```python
from build123d import *

# Parameters (mm, degrees)
SKETCH1_W           = 230
SKETCH1_H           = 90
SKETCH1_R           = 5
SKETCH1_R_2         = 3.5
SKETCH1_R_3         = 2.25
SKETCH1_W_2         = 40
SKETCH1_H_2         = 10
SKETCH1_H_3         = 7
BOSS_EXTRUDE1_DEPTH = 6
SKETCH2_W           = 230
SKETCH2_H           = 6
BOSS_EXTRUDE2_DEPTH = 12
CUT_EXTRUDE1_REACH  = 145.544
SKETCH3_R           = 2.25


with BuildPart() as part:
    # Sketch1 → Boss-Extrude1 (new body)
    with BuildSketch(Plane(origin=(0, 0, 0), x_dir=(1, 0, 0), z_dir=(0, 1, 0))):
        Rectangle(SKETCH1_W, SKETCH1_H)
        with Locations(Location((0, 0, 0), (0, 0, 270))):
            Circle(SKETCH1_R, mode=Mode.SUBTRACT)
        with Locations(Location((0, 22.25, 0), (0, 0, 270))):
            Circle(SKETCH1_R_2, mode=Mode.SUBTRACT)
        with Locations(Location((0, -22.25, 0), (0, 0, 90))):
            Circle(SKETCH1_R_2, mode=Mode.SUBTRACT)
        with Locations(Location((110, 40, 0), (0, 0, 270))):
            Circle(SKETCH1_R_3, mode=Mode.SUBTRACT)
        with Locations(Location((110, -32.5, 0), (0, 0, 270))):
            Circle(SKETCH1_R_3, mode=Mode.SUBTRACT)
        with Locations(Location((-110, 40, 0), (0, 0, 90))):
            Circle(SKETCH1_R_3, mode=Mode.SUBTRACT)
        with Locations(Location((-110, -32.5, 0), (0, 0, 90))):
            Circle(SKETCH1_R_3, mode=Mode.SUBTRACT)
        with Locations((55, 0)):
            Rectangle(SKETCH1_W_2, SKETCH1_H_2, mode=Mode.SUBTRACT)
        with Locations((55, 22.25)):
            Rectangle(SKETCH1_W_2, SKETCH1_H_3, mode=Mode.SUBTRACT)
        with Locations((55, -22.25)):
            Rectangle(SKETCH1_W_2, SKETCH1_H_3, mode=Mode.SUBTRACT)
        with Locations((-55, -22.25)):
            Rectangle(SKETCH1_W_2, SKETCH1_H_3, mode=Mode.SUBTRACT)
        with Locations((-55, 0)):
            Rectangle(SKETCH1_W_2, SKETCH1_H_2, mode=Mode.SUBTRACT)
        with Locations((-55, 22.25)):
            Rectangle(SKETCH1_W_2, SKETCH1_H_3, mode=Mode.SUBTRACT)
    extrude(amount=BOSS_EXTRUDE1_DEPTH)

    # Sketch2 → Boss-Extrude2 (add)
    with BuildSketch(Plane(origin=(0, 6, 0), x_dir=(1, 0, 0), z_dir=(0, 1, 0))):
        with Locations((0, -42)):
            Rectangle(SKETCH2_W, SKETCH2_H)
    extrude(amount=BOSS_EXTRUDE2_DEPTH)

    # Sketch3 → Cut-Extrude1 (cut, up to next)
    with BuildSketch(Plane(origin=(0, 0, 39), x_dir=(-1, 0, 0), z_dir=(0, 0, -1)), mode=Mode.PRIVATE) as cut_extrude1_sk1:
        with Locations((0, 12)):
            Circle(SKETCH3_R)
    cut_extrude1_tool1 = extrude(cut_extrude1_sk1.sketch, amount=-CUT_EXTRUDE1_REACH, mode=Mode.PRIVATE) & part.part
    # Sketch3 → Cut-Extrude1 (cut, up to next)
    with BuildSketch(Plane(origin=(0, 0, 39), x_dir=(-1, 0, 0), z_dir=(0, 0, -1)), mode=Mode.PRIVATE) as cut_extrude1_sk2:
        with Locations((100, 12)):
            Circle(SKETCH3_R)
    cut_extrude1_tool2 = extrude(cut_extrude1_sk2.sketch, amount=-CUT_EXTRUDE1_REACH, mode=Mode.PRIVATE) & part.part
    # Sketch3 → Cut-Extrude1 (cut, up to next)
    with BuildSketch(Plane(origin=(0, 0, 39), x_dir=(-1, 0, 0), z_dir=(0, 0, -1)), mode=Mode.PRIVATE) as cut_extrude1_sk3:
        with Locations((-100, 12)):
            Circle(SKETCH3_R)
    cut_extrude1_tool3 = extrude(cut_extrude1_sk3.sketch, amount=-CUT_EXTRUDE1_REACH, mode=Mode.PRIVATE) & part.part
    add(cut_extrude1_tool1.solids().sort_by_distance((0, 12, 39))[0], mode=Mode.SUBTRACT)
    add(cut_extrude1_tool2.solids().sort_by_distance((-100, 12, 39))[0], mode=Mode.SUBTRACT)
    add(cut_extrude1_tool3.solids().sort_by_distance((100, 12, 39))[0], mode=Mode.SUBTRACT)


solid = part.part
```
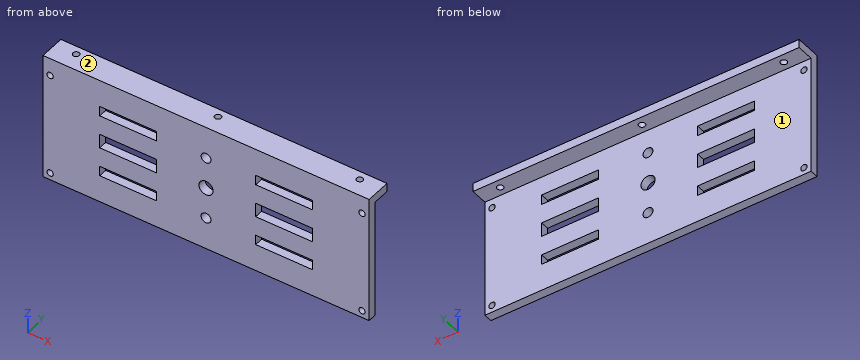
CAD build for the part. Positions are in the model's coordinates, mm. Face numbers are marked on the shaded views. A direction names the side the tool comes from. Round coordinates to 2 decimals unless told otherwise and drop trailing zeros. Order: outer loops, then holes, each group sorted by start corner. A loop starts at its lowest first (then second) coordinate and runs counter-clockwise, first axis right, second up.
Item 1: Saw through at C-C on z = 32.5. Write the cut outline in (x, y), then the cut area to 3 significant figures.
Item 2: Tool access for the marked faces 1 and 2: list every direction of +Z, -Z, +X, -X, +Y, -Y with a clear straight run to the whole face (end or side of a thin tool).
Item 3: Saw through at D-D on x = 110. Write the cut outline in (y, z).
Item 4: Saw through at A-A on x = -100. Write the cut outline in (y, z).
Item 5: Pin check, flat tips, straight feed: pin 1 (4 mm diameter, centred on x = 0, y = 12, fed in from +Z); pin 2 (5 mm diameter, centred on x = -110, z = 32.5, fed in from +Y). Stop position of each tip, or through.
Item 6: Probe line 1 along Z through (x, y) = (-110, 2.55); line 2 along X through (y, z) = (1.4, 0); line 3 along Y through (x, z) = (0, 42.7). List the from-to ranges inside material, lowest first.
Item 7: Saw through at B-B on z = 22.25. Write the cut outline in (x, y).
Reported:
1. outline: (-115, 0) - (-112.25, 0) - (-112.25, 6) - (-115, 6) - close; (-107.75, 0) - (107.75, 0) - (107.75, 6) - (-107.75, 6) - close; (112.25, 0) - (115, 0) - (115, 6) - (112.25, 6) - close
1. area: 1,330 mm2
2. face 1: -Z, +X, -X, +Y
2. face 2: +Z, +X, -X, +Y, -Y
3. outline: (0, -45) - (6, -45) - (6, -42.25) - (0, -42.25) - close; (0, -37.75) - (6, -37.75) - (6, 30.25) - (0, 30.25) - close; (0, 34.75) - (6, 34.75) - (6, 39) - (18, 39) - (18, 45) - (0, 45) - close
4. outline: (0, -45) - (6, -45) - (6, 39) - (9.75, 39) - (9.75, 45) - (0, 45) - close; (14.25, 39) - (18, 39) - (18, 45) - (14.25, 45) - close
5. pin 1: passes through
5. pin 2: stops at y = 6
6. line 1: z = -45 to -42.25, -37.75 to 30.25, 34.75 to 45
6. line 2: x = -115 to -75, -35 to -5, 5 to 35, 75 to 115
6. line 3: y = 0 to 9.75, 14.25 to 18
7. outline: (-115, 0) - (-75, 0) - (-75, 6) - (-115, 6) - close; (-35, 0) - (-3.5, 0) - (-3.5, 6) - (-35, 6) - close; (3.5, 0) - (35, 0) - (35, 6) - (3.5, 6) - close; (75, 0) - (115, 0) - (115, 6) - (75, 6) - close
